Here's how the part is built. I have some questions about the finished solid (model axes, mm). A direction names the side the tool comes from. Give positions to 0.01 mm unless a question says otherwise; leave off trailing zeros. Loops run counter-clockwise (first coordinate to the right, second up) from the corner with the lowest first, then second, coordinate; pieces in that order, holes last. Notation, with made-up numbers: (-30.75, 81.5) - (21.25, 81.5) arc R12 cw to (21.25, 103.5) - close; hole circle Ø5 at (-29.5, 77). An arc over 180 degrees is marked (long way). Use a Markdown table: item, result.
from build123d import *

# Parameters (mm, degrees)
F0_W         = 203.2
F0_H         = 101.6
F1_DEPTH     = 50.8
F2_R         = 5.08
F3_SIZE      = 38.1
F4_T1_DEPTH  = 71.12
F4_T3_DEPTH  = 58.42
F4_T6_ANGLE  = 90
F5_R         = 5.08
F6_T1_DEPTH  = 64.4773318296
F6_T3_DEPTH  = 193.04
F6_T8_DEPTH  = 5.08
F6_T14_DEPTH = 5.08
F7_T1_DEPTH  = 193.04
F7_T3_DEPTH  = 23.2957951031
F7_T8_DEPTH  = 5.08
F7_T14_DEPTH = 5.08
F8_W         = 104.7176718712
F8_H         = 41.105248034
F9_DEPTH     = 6.35
F10_R        = 10.900008085
F11_DEPTH    = 76.2
F12_W        = 83.9344151318
F12_H        = 34.3853458762
F13_DEPTH    = 25.4


# Not quite as in the source:
# - a fillet or chamfer that OpenCascade refuses, or shapes differently, is made with other operations: its cross-section is extruded or revolved along the edge and cut away or added


with BuildPart() as f1:
    # F0 (on Front) → F1 (new body)
    with BuildSketch(Plane.XZ):
        Rectangle(F0_W, F0_H)
    extrude(amount=F1_DEPTH)

    # F2
    f2_edges = [f1.edges().sort_by_distance(p)[0] for p in [
        (0, 0, -50.8),
    ]]
    fillet(f2_edges, radius=F2_R)

    # F3
    f3_edges = [f1.edges().sort_by_distance(p)[0] for p in [
        (0, 0, 50.8),
    ]]
    chamfer(f3_edges, length=F3_SIZE)

    # F4: fillet of radius 5.08 on 1 edges, made by hand

    # F4_s2 → F4_t1 (cut)
    with BuildSketch(Plane.XY.offset(-45.72)):
        with BuildLine():
            ThreePointArc((-101.6, -5.08), (-100.1121024484, -1.4878975516), (-96.52, 0))
            Line((-96.52, 0), (-101.6, 0))
            Line((-101.6, 0), (-101.6, -5.08))
        make_face()
    extrude(amount=F4_T1_DEPTH, mode=Mode.SUBTRACT)

    # F4_s4 → F4_t3 (cut)
    with BuildSketch(Plane.XZ.offset(5.08)):
        with BuildLine():
            ThreePointArc((-101.6, -45.72), (-100.1121024484, -49.3121024484), (-96.52, -50.8))
            Line((-96.52, -50.8), (-101.6, -50.8))
            Line((-101.6, -50.8), (-101.6, -45.72))
        make_face()
    extrude(amount=F4_T3_DEPTH, mode=Mode.SUBTRACT)

    # F4_s5 → F4_t6 (revolve, cut)
    with BuildSketch(Plane.XZ.offset(5.08)):
        with BuildLine():
            ThreePointArc((-101.6, -45.72), (-100.1121024484, -49.3121024484), (-96.52, -50.8))
            Line((-96.52, -50.8), (-101.6, -50.8))
            Line((-101.6, -50.8), (-101.6, -45.72))
        make_face()
    revolve(axis=Axis((-101.6, -5.08, -45.72), (1, 0, 0)), revolution_arc=F4_T6_ANGLE, mode=Mode.SUBTRACT)

    # F5
    f5_edges = [f1.edges().sort_by_distance(p)[0] for p in [
        (101.6, 0, -16.51),
    ]]
    fillet(f5_edges, radius=F5_R)

    # F6: fillet of radius 5.08 on 1 edges, made by hand

    # F6_s2 → F6_t1 (cut)
    with BuildSketch(Plane(origin=(0, -7.8378975516, 7.8378975516), x_dir=(1, 0, 0), z_dir=(0, -0.7071067812, 0.7071067812))):
        with BuildLine():
            ThreePointArc((101.6, 3.9002561211), (100.1121024484, 7.4923585695), (96.52, 8.9802561211))
            Line((96.52, 8.9802561211), (101.6, 8.9802561211))
            Line((101.6, 8.9802561211), (101.6, 3.9002561211))
        make_face()
        with BuildLine():
            ThreePointArc((-101.6, 3.9002561211), (-100.1121024484, 7.4923585695), (-96.52, 8.9802561211))
            Line((-96.52, 8.9802561211), (-101.6, 8.9802561211))
            Line((-101.6, 8.9802561211), (-101.6, 3.9002561211))
        make_face()
    extrude(amount=F6_T1_DEPTH, mode=Mode.SUBTRACT)

    # F6_s4 → F6_t3 (cut)
    with BuildSketch(Plane.YZ.offset(-96.52)):
        with BuildLine():
            ThreePointArc((0, 10.5957951031), (-0.3866919748, 12.5398269396), (-1.4878975516, 14.1878975516))
            Line((-1.4878975516, 14.1878975516), (0, 12.7))
            Line((0, 12.7), (0, 10.5957951031))
        make_face()
    extrude(amount=F6_T3_DEPTH, mode=Mode.SUBTRACT)


with BuildPart() as f6_tool6:
    # F6_s7 → F6_t8 (new body)
    with BuildSketch(Plane.YZ.offset(96.52)):
        Polygon((-5.08, 10.5957951031), (-1.4878975516, 14.1878975516), (0, 12.7), (0, 10.5957951031), align=None)
    extrude(amount=F6_T8_DEPTH)

    # F6_s9 → F6_t10 (revolve, cut)
    with BuildSketch(Plane(origin=(96.52, -5.08, 10.5957951031), x_dir=(0, -0.9238795325, -0.3826834324), z_dir=(0, -0.3826834324, 0.9238795325))):
        with BuildLine():
            ThreePointArc((0, -5.08), (5.08, 0), (0, 5.08))
            Line((0, 5.08), (0, -5.08))
        make_face()
    revolve(axis=Axis((96.52, -5.08, 10.5957951031), (1, 0, 0)), mode=Mode.SUBTRACT)


with BuildPart() as f1_1:
    add(f1.part)

    # F6_t5: cut F6_tool6
    add(f6_tool6.part, mode=Mode.SUBTRACT)


with BuildPart() as f6_tool12:
    # F6_s13 → F6_t14 (new body)
    with BuildSketch(Plane.YZ.offset(-96.52)):
        Polygon((-5.08, 10.5957951031), (-1.4878975516, 14.1878975516), (0, 12.7), (0, 10.5957951031), align=None)
    extrude(amount=-F6_T14_DEPTH)

    # F6_s15 → F6_t16 (revolve, cut)
    with BuildSketch(Plane(origin=(-96.52, -5.08, 10.5957951031), x_dir=(0, -0.9238795325, -0.3826834324), z_dir=(0, 0.3826834324, -0.9238795325))):
        with BuildLine():
            ThreePointArc((0, -5.08), (5.08, 0), (0, 5.08))
            Line((0, 5.08), (0, -5.08))
        make_face()
    revolve(axis=Axis((-96.52, -5.08, 10.5957951031), (-1, 0, 0)), mode=Mode.SUBTRACT)


with BuildPart() as f1_2:
    add(f1_1.part)

    # F6_t11: cut F6_tool12
    add(f6_tool12.part, mode=Mode.SUBTRACT)

    # F7: fillet of radius 5.08 on 3 edges, made by hand

    # F7_s2 → F7_t1 (cut)
    with BuildSketch(Plane.YZ.offset(-96.52)):
        with BuildLine():
            ThreePointArc((-40.2042048969, 50.8), (-38.2601730604, 50.4133080252), (-36.6121024484, 49.3121024484))
            Line((-36.6121024484, 49.3121024484), (-38.1, 50.8))
            Line((-38.1, 50.8), (-40.2042048969, 50.8))
        make_face()
    extrude(amount=F7_T1_DEPTH, mode=Mode.SUBTRACT)

    # F7_s4 → F7_t3 (cut)
    with BuildSketch(Plane.XZ.offset(40.2042048969)):
        with BuildLine():
            ThreePointArc((101.6, 45.72), (100.1121024484, 49.3121024484), (96.52, 50.8))
            Line((96.52, 50.8), (101.6, 50.8))
            Line((101.6, 50.8), (101.6, 45.72))
        make_face()
        with BuildLine():
            ThreePointArc((-101.6, 45.72), (-100.1121024484, 49.3121024484), (-96.52, 50.8))
            Line((-96.52, 50.8), (-101.6, 50.8))
            Line((-101.6, 50.8), (-101.6, 45.72))
        make_face()
    extrude(amount=F7_T3_DEPTH, mode=Mode.SUBTRACT)


with BuildPart() as f7_tool6:
    # F7_s7 → F7_t8 (new body)
    with BuildSketch(Plane.YZ.offset(-96.52)):
        Polygon((-40.2042048969, 45.72), (-40.2042048969, 50.8), (-38.1, 50.8), (-36.6121024484, 49.3121024484), align=None)
    extrude(amount=-F7_T8_DEPTH)

    # F7_s9 → F7_t10 (revolve, cut)
    with BuildSketch(Plane(origin=(-96.52, -40.2042048969, 45.72), x_dir=(0, -0.3826834324, -0.9238795325), z_dir=(0, 0.9238795325, -0.3826834324))):
        with BuildLine():
            ThreePointArc((0, -5.08), (5.08, 0), (0, 5.08))
            Line((0, 5.08), (0, -5.08))
        make_face()
    revolve(axis=Axis((-96.52, -40.2042048969, 45.72), (-1, 0, 0)), mode=Mode.SUBTRACT)


with BuildPart() as f1_3:
    add(f1_2.part)

    # F7_t5: cut F7_tool6
    add(f7_tool6.part, mode=Mode.SUBTRACT)


with BuildPart() as f7_tool12:
    # F7_s13 → F7_t14 (new body)
    with BuildSketch(Plane.YZ.offset(96.52)):
        Polygon((-40.2042048969, 45.72), (-40.2042048969, 50.8), (-38.1, 50.8), (-36.6121024484, 49.3121024484), align=None)
    extrude(amount=F7_T14_DEPTH)

    # F7_s15 → F7_t16 (revolve, cut)
    with BuildSketch(Plane(origin=(96.52, -40.2042048969, 45.72), x_dir=(0, -0.3826834324, -0.9238795325), z_dir=(0, -0.9238795325, 0.3826834324))):
        with BuildLine():
            ThreePointArc((0, -5.08), (5.08, 0), (0, 5.08))
            Line((0, 5.08), (0, -5.08))
        make_face()
    revolve(axis=Axis((96.52, -40.2042048969, 45.72), (1, 0, 0)), mode=Mode.SUBTRACT)


with BuildPart() as f1_4:
    add(f1_3.part)

    # F7_t11: cut F7_tool12
    add(f7_tool12.part, mode=Mode.SUBTRACT)

    # F8 (on face) → F9 (join)
    with BuildSketch(Plane(origin=(0, 0, 0), x_dir=(-1, 0, 0), z_dir=(0, 1, 0))):
        with Locations((0, -17.4928158522)):
            Rectangle(F8_W, F8_H)
    extrude(amount=F9_DEPTH)

    # F10 (on face) → F11 (join)
    with BuildSketch(Plane(origin=(0, 6.35, 0), x_dir=(-1, 0, 0), z_dir=(0, 1, 0))):
        with Locations((-18.5013078153, -16.3395497948)):
            Circle(F10_R)
        with Locations((20.8696890622, -17.3914972693)):
            Circle(F10_R)
    extrude(amount=F11_DEPTH)

    # F12 (on face) → F13 (join)
    with BuildSketch(Plane(origin=(0, 82.55, 0), x_dir=(-1, 0, 0), z_dir=(0, 1, 0))):
        with Locations((0.4271473736, -17.1926729381)):
            Rectangle(F12_W, F12_H)
    extrude(amount=F13_DEPTH)


solid = f1_4.part
(1) Suppose I cut it at D-D on y = 74.5. Write out the boundary of the cut face in (x, z).
A:
| item | result |
|---|---|
| outline | circle Ø21.8 at (-20.87, -17.39); circle Ø21.8 at (18.5, -16.34) |
(2) Will these pins go through, and if not, where does the flat tip stop? pin 1 (7.5 mm diameter, centred on x = 0, y = 97, fed in from -Z); pin 2 (20.5 mm diameter, centred on y = 101, z = -21.5, fed in from +X); pin 3 (10 mm diameter, centred on x = -74.5, y = -6, fed in from +Z).
A:
| item | result |
|---|---|
| pin 1 | z = -34.39 |
| pin 2 | x = 41.54 |
| pin 3 | z = 23.7 |
(3) Suppose I cut it at B-B on z = -10.5. Write out the boundary of the cut face in (x, y).
A:
| item | result |
|---|---|
| outline | (-101.6, -50.8) - (101.6, -50.8) - (101.6, -5.08) arc R5.08 ccw to (96.52, 0) - (52.36, 0) - (52.36, 6.35) - (27.71, 6.35) - (27.71, 82.55) - (41.54, 82.55) - (41.54, 107.95) - (-42.39, 107.95) - (-42.39, 82.55) - (-29.31, 82.55) - (-29.31, 6.35) - (-52.36, 6.35) - (-52.36, 0) - (-96.52, 0) arc R5.08 ccw to (-101.6, -5.08) - close; hole (-12.42, 6.35) - (9.3, 6.35) - (9.3, 82.55) - (-12.42, 82.55) - close |
(4) If I drill on line 1 (Y direction, x = 39, z = -2); line 2 (Y direction, x = 71.5, z = -6); line 3 (X direction, y = 95.5, z = -2), over which ranges is the centre line in solid material (lowest first)?
A:
| item | result |
|---|---|
| line 1 | -50.8 to 6.35, 82.55 to 107.95 |
| line 2 | -50.8 to 0 |
| line 3 | -42.39 to 41.54 |
(5) Suppose I cut it at A-A on x = 3.5. Write out the boundary of the cut face in (y, z), plus the area to 3 significant figures.
A:
| item | result |
|---|---|
| outline | (-50.8, -50.8) - (-5.08, -50.8) arc R5.08 ccw to (0, -45.72) - (0, -38.05) - (6.35, -38.05) - (6.35, 3.06) - (0, 3.06) - (0, 10.6) arc R5.08 ccw to (-1.49, 14.19) - (-36.61, 49.31) arc R5.08 ccw to (-40.2, 50.8) - (-50.8, 50.8) - close; (82.55, -34.39) - (107.95, -34.39) - (107.95, 0) - (82.55, 0) - close |
| area | 5,560 mm2 |
(6) We'd pull the mould along X, two halves only. Please class faces 4 (the face through (-9.98, 43.92, -16.91)), 5 (the face through (0, 95, -34.385)), 6 (the face through (100.151, -45.428, 49.272)), 7 (the face through (-100.15, -19.88, 30.42)): pulls with the +X half, pulls with the -X half, needs draft (parallel to the pull), parting line crosses it, or undercut.
A:
| item | result |
|---|---|
| face 4 | undercut |
| face 5 | needs draft |
| face 6 | pulls with the +X half |
| face 7 | pulls with the -X half |
(7) Suppose I cut it at C-C on x = -83.5. Write out the boundary of the cut face in (y, z), plus the area to 3 significant figures.
A:
| item | result |
|---|---|
| outline | (-50.8, -50.8) - (-5.08, -50.8) arc R5.08 ccw to (0, -45.72) - (0, 10.6) arc R5.08 ccw to (-1.49, 14.19) - (-36.61, 49.31) arc R5.08 ccw to (-40.2, 50.8) - (-50.8, 50.8) - close |
| area | 4,430 mm2 |
(8) On a 3-axis mill with a long thin cutter (end or side, diameter ignored), from which of +Z, -Z, +X, -X, +Y, -Y can I reach the whole of each face in a straight line? I mean faces 1 (the face through (0, 95, 0)), 2 (the face through (41.54, 95, -17)), 3 (the face through (1, 6.35, -17)). Say none if no direction works.
A:
| item | result |
|---|---|
| face 1 | +Z, +X, -X, +Y |
| face 2 | +Z, -Z, +X, +Y |
| face 3 | none |
